The drawing under review shows one solid part. Ordinate dimensions are in mm from its lowest x, y, z. A direction names the side the tool comes from. Round coordinates to 2 decimals unless told otherwise and drop trailing zeros. Write each loop counter-clockwise with the first axis right and the second up, starting at its lowest first coordinate (ties: lowest second). Pieces come first, ordered by that corner, then holes. Notation, with made-up numbers: M 40.5,32 L 96.5,32 A14 ccw 96.5,53 Z; hole C -14,53 d5. An arc over 180 degrees is marked long. One line per item, written item: value. Start each with the question number.
1) For P1, Ø4, axis at x = 30, y = 4.5, coming from the -Z side; P2, Ø8, axis at x = 15.5, y = 14, coming from the -Z side; P3, Ø7.5, axis at y = 22.5, z = 34.5, coming from the +X side; P4, Ø12, axis at x = 18.5, y = 12.5, coming from the +Z side (1 decimal), all flat-tipped, find the tip position at first contact; note any pin that passes through.
2) Wall thickness on probe 1 along Z at (x, y) = (28.5, 3) (1 decimal); probe 2 along X at (y, z) = (6.5, 8); probe 3 along Z at (x, y) = (34, 4.5) (1 decimal): over which ranges is each line inside the solid? List them lowest first.
3) Tool access review of the marked faces 1, 2, 3, 4 and 5: name each direction out of +Z, -Z, +X, -X, +Y, -Y from which nothing blocks a thin tool from reaching the whole face with its end or side.
4) Mouldability with a two-part tool opening along Z and no side actions: class the marked faces 6, 7 and 8 as +Z half, -Z half, draft (parallel to the pull), parting line (faces both ways), or undercut.
5) Take a section at C-C, the plane z = 38. Write out the cut boundary in (x, y).
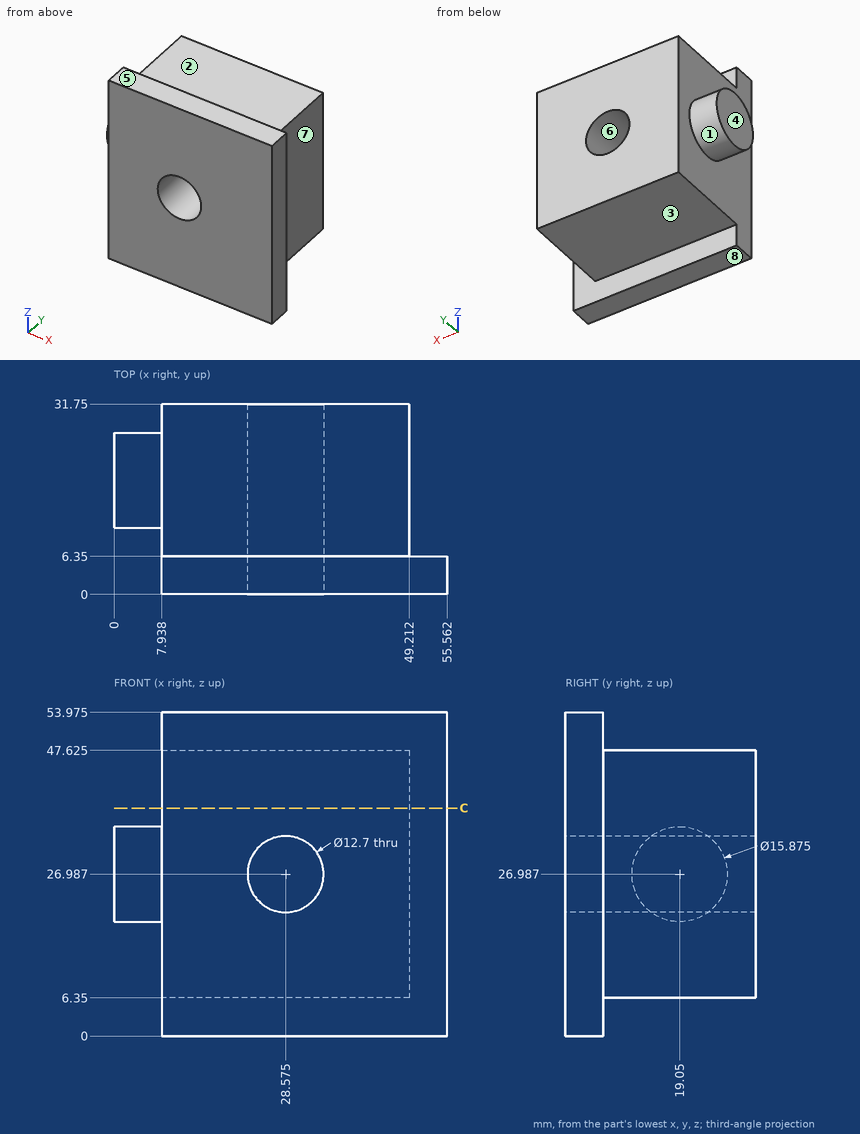
Checked values:
1. P1: stops at z = 0
1. P2: stops at z = 6.35
1. P3: stops at x = 49.21
1. P4: stops at z = 47.6
2. probe 1: z = 0 to 20.6, 33.3 to 54
2. probe 2: x = 7.94 to 49.21
2. probe 3: z = 0 to 23.7, 30.3 to 54
3. face 1: -X
3. face 2: +Z, +X, -X, +Y
3. face 3: -Z, +X, -X, +Y
3. face 4: +Z, -Z, -X, +Y, -Y
3. face 5: +Z, +X, -X, +Y, -Y
4. face 6: undercut
4. face 7: draft
4. face 8: -Z half
5. outline: M 7.94,0 L 55.56,0 L 55.56,6.35 L 49.21,6.35 L 49.21,31.75 L 7.94,31.75 Z
